Check sheet for the drawn part. Datum: minimum x, y, z corner. Units: mm. Coordinates: 2 decimals unless noted, no trailing zeros. Loops run counter-clockwise (first coordinate to the right, second up) from the corner with the lowest first, then second, coordinate; pieces in that order, holes last.
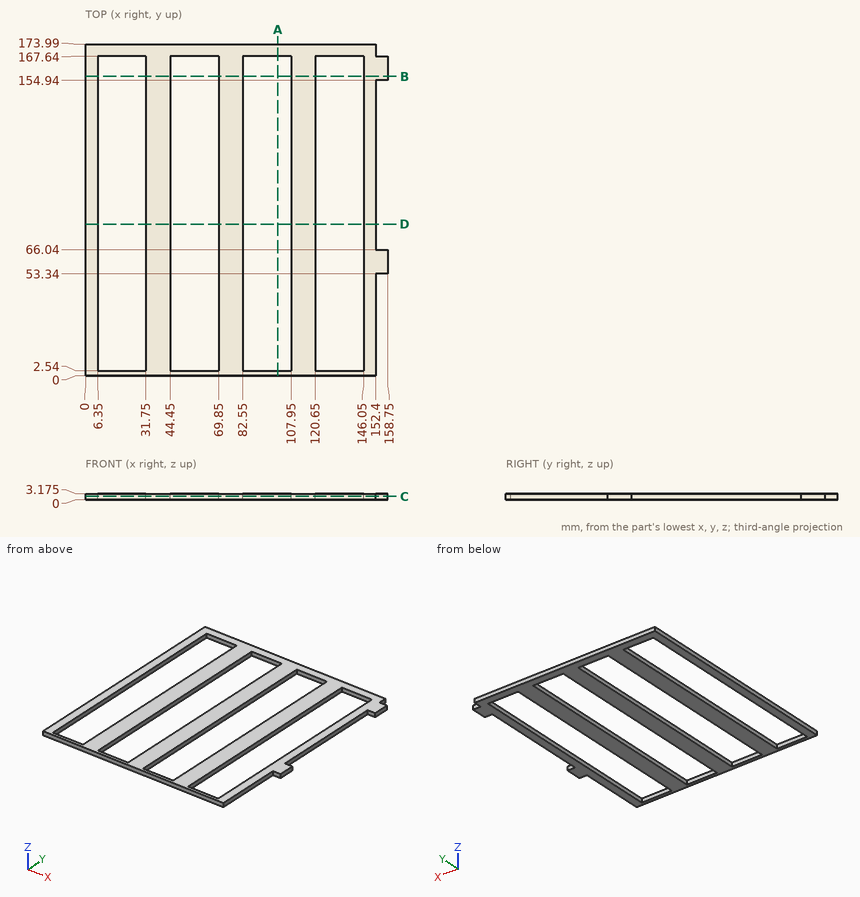
(1) Sectioned sample at A-A on x = 101. Record the cut outline in (y, z) (3 decimals).
Findings:
outline: (0, 0) - (2.54, 0) - (2.54, 3.175) - (0, 3.175) - close; (167.64, 0) - (173.99, 0) - (173.99, 3.175) - (167.64, 3.175) - close
(2) Sectioned sample at D-D on y = 79.5. Record the cut outline in (x, z) (3 decimals), and give its area (3 significant figures).
Findings:
outline: (0, 0) - (6.35, 0) - (6.35, 3.175) - (0, 3.175) - close; (31.75, 0) - (44.45, 0) - (44.45, 3.175) - (31.75, 3.175) - close; (69.85, 0) - (82.55, 0) - (82.55, 3.175) - (69.85, 3.175) - close; (107.95, 0) - (120.65, 0) - (120.65, 3.175) - (107.95, 3.175) - close; (146.05, 0) - (152.4, 0) - (152.4, 3.175) - (146.05, 3.175) - close
area: 161 mm2
(3) Scan lines: L1, parallel to X at y = 131, z = 0.55; L2, parallel to X at y = 55, z = 0.5; L3, parallel to Y at x = 101, z = 1.65. Record each from-to range of solid material in increasing order.
Findings:
L1: x = 0 to 6.35, 31.75 to 44.45, 69.85 to 82.55, 107.95 to 120.65, 146.05 to 152.4
L2: x = 0 to 6.35, 31.75 to 44.45, 69.85 to 82.55, 107.95 to 120.65, 146.05 to 158.75
L3: y = 0 to 2.54, 167.64 to 173.99
(4) Gauge pin test, flat ends, axial feed: pin 1 Ø1 at (y, z) = (111, 1.5) entering from +X; pin 2 Ø1.5 at (x, y) = (83.5, 152.5) entering from +Z. Record the tip position at first contact, or that the pin passes through.
Findings:
pin 1: stops at x = 152.4
pin 2: passes through
(5) Sectioned sample at B-B on y = 157. Record the cut outline in (x, z) (3 decimals).
Findings:
outline: (0, 0) - (6.35, 0) - (6.35, 3.175) - (0, 3.175) - close; (31.75, 0) - (44.45, 0) - (44.45, 3.175) - (31.75, 3.175) - close; (69.85, 0) - (82.55, 0) - (82.55, 3.175) - (69.85, 3.175) - close; (107.95, 0) - (120.65, 0) - (120.65, 3.175) - (107.95, 3.175) - close; (146.05, 0) - (158.75, 0) - (158.75, 3.175) - (146.05, 3.175) - close
(6) Sectioned sample at C-C on z = 1.65. Record the cut outline in (x, y), and give its area (3 significant figures).
Findings:
outline: (0, 0) - (152.4, 0) - (152.4, 53.34) - (158.75, 53.34) - (158.75, 66.04) - (152.4, 66.04) - (152.4, 154.94) - (158.75, 154.94) - (158.75, 167.64) - (152.4, 167.64) - (152.4, 173.99) - (0, 173.99) - close; hole (6.35, 2.54) - (31.75, 2.54) - (31.75, 167.64) - (6.35, 167.64) - close; hole (44.45, 2.54) - (69.85, 2.54) - (69.85, 167.64) - (44.45, 167.64) - close; hole (82.55, 2.54) - (107.95, 2.54) - (107.95, 167.64) - (82.55, 167.64) - close; hole (120.65, 2.54) - (146.05, 2.54) - (146.05, 167.64) - (120.65, 167.64) - close
area: 9,900 mm2
